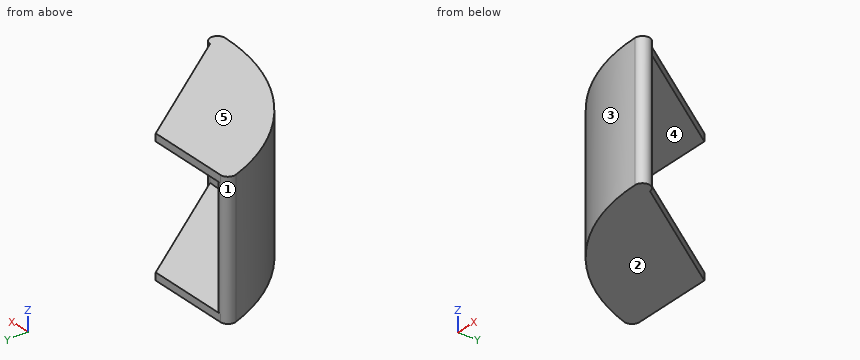
from build123d import *

# Parameters (mm, degrees)
BASE_DEPTH         = 90
WALL_DEPTH         = 10
CUT_EXTRUDE2_DEPTH = 181


with BuildPart() as part:
    # Sketch1 → Base (new body, symmetric)
    with BuildSketch(Plane.XY):
        with BuildLine():
            ThreePointArc((-9.513513741, 156.91891962), (78.103574675, 36.142415178), (220.000000737, -10))
            ThreePointArc((220.000000737, -10), (230, 7.37e-07), (219.999999263, 10))
            ThreePointArc((219.999999263, 10), (89.867008629, 52.317136864), (9.513513741, 163.08108038))
            ThreePointArc((9.513513741, 163.08108038), (-3.08108038, 169.513513741), (-9.513513741, 156.91891962))
        make_face()
    extrude(amount=BASE_DEPTH, both=True)

    # Sketch3 → Wall (add)
    with BuildSketch(Plane.XY.offset(80)):
        with BuildLine():
            Line((0, 170), (219.999999263, 170))
            Line((219.999999263, 170), (219.999999263, 10))
            ThreePointArc((219.999999263, 10), (89.867008629, 52.317136864), (9.513513741, 163.08108038))
            ThreePointArc((9.513513741, 163.08108038), (5.881717275, 168.087360626), (0, 170))
        make_face()
    wall = extrude(amount=WALL_DEPTH)

    # Mirror4: Wall across plane
    add(wall.mirror(Plane(origin=(0, 0, 0), x_dir=(1, 0, 0), z_dir=(0, 0, -1))))

    # Sketch5 → Cut-Extrude2 (cut, through all)
    with BuildSketch(Plane.XY.offset(90)):
        Polygon((219.999999263, 10), (109.999999631, 170), (219.999999263, 170), align=None)
    extrude(amount=-CUT_EXTRUDE2_DEPTH, mode=Mode.SUBTRACT)


solid = part.part
Read the model definition and answer for the solid it produces. Units are mm, in the model's axes. Face numbers are marked on the shaded views. A direction names the side the tool comes from. Give positions to 0.01 mm unless a question says otherwise; leave off trailing zeros. Write each loop counter-clockwise with the first axis right and the second up, starting at its lowest first coordinate (ties: lowest second). Pieces come first, ordered by that corner, then holes. Notation, with made-up numbers: (7, 78) - (16, 78) arc R17 ccw to (16, 94) - close; hole circle Ø6 at (75, -14). An arc over 180 degrees is marked (long way). Use CSV: the item, a comma, the result in double quotes. Start each with the question number.
(1) Find section C-C (z = 57). Give the vertices of the cut face in (x, y), plus the area to 3 significant figures.
(2) Find section D-D (y = 0). Give the vertices of the cut face in (x, z).
(3) Given P1, Ø12, axis at y = 25.5, z = -70, coming from the -X side; P2, Ø12, axis at y = 111, z = 51.5, coming from the +X side; P3, Ø1.5, axis at x = 67, z = -39, coming from the +Y side, each flat-ended and moving along its own axis, determine where each tip first touches the part or whether it passes through.
(4) Find section B-B (x = 85.5). Give the vertices of the cut face in (y, z), plus the area to 3 significant figures.
(5) Determine the mould class of the marked faces 1, 2 and 3 for opening direction Z: +Z half, -Z half, draft (parallel to the pull), parting line (faces both ways), or undercut.
(6) Find section A-A (y = 160). Give the vertices of the cut face in (x, z) (3 decimals).
(7) Consider line 1 along Z through (x, y) = (113, 110); line 2 along Y through (x, z) = (49.5, -14.5); line 3 along Y through (x, z) = (70.5, 26). Determine where each line is inside the solid, lowest interval first.
(8) For the marked faces 4 and 5, determine the directions among +Z, -Z, +X, -X, +Y, -Y from which every point of the face is accessible in a straight line to the end or side of a thin tool.
Findings below:
1,outline,"(-9.51, 156.92) arc R241.25 ccw to (220, -10) arc R10 ccw to (220, 10) arc R221.25 cw to (9.51, 163.08) arc R10 ccw to start"
1,area,"6,130 mm2"
2,outline,"(151.26, -90) - (230, -90) - (230, 90) - (151.26, 90) - close"
3,P1,"x = 84.72"
3,P2,"x = 38.31"
3,P3,"y = 72.15"
4,outline,"(30.97, -90) - (170, -90) - (170, -80) - (55.58, -80) - (55.58, 80) - (170, 80) - (170, 90) - (30.97, 90) - close"
4,area,"6,720 mm2"
5,face 1,"undercut"
5,face 2,"-Z half"
5,face 3,"draft"
6,outline,"(-10, -90) - (116.875, -90) - (116.875, -80) - (10.536, -80) - (10.536, 80) - (116.875, 80) - (116.875, 90) - (-10, 90) - close"
7,line 1,"-90 to -80, 80 to 90"
7,line 2,"60.57 to 90.25"
7,line 3,"41.91 to 68.15"
8,face 4,"+X, +Y"
8,face 5,"+Z, +X, -X, +Y, -Y"
